Here's how the part is built. I have some questions about the finished solid (model axes, mm). Face numbers are marked on the shaded views. A direction names the side the tool comes from. Round coordinates to 2 decimals unless told otherwise and drop trailing zeros. Write each loop counter-clockwise with the first axis right and the second up, starting at its lowest first coordinate (ties: lowest second). Pieces come first, ordered by that corner, then holes. Notation, with made-up numbers: (82.25, 30) -> (126.25, 30) arc R9 ccw to (126.25, 39) -> close; hole circle Ø1 at (36, 64). An arc over 180 degrees is marked (long way). Put each result on its own line as item: value. Start each with the question number.
1. Suppose I cut it at D-D (z = 27). Count the separate pieces of the cut face and the enclosed holes in it, then the cut area to 3 significant figures.
2. Which directions (+Z, -Z, +X, -X, +Y, -Y) give clear straight access to the entire face, cutting with the end or side of a thin tool? Please do the marked faces 1 and 2.
3. Suppose I cut it at C-C (z = 7). Please give me the cut outline in (x, y), then the cut area to 3 significant figures.
4. Suppose I cut it at A-A (y = 0). Please give me the cut outline in (x, z), then the cut area to 3 significant figures.
5. For pin 1 (1.4 mm diameter, centred on x = -42, z = 27, fed in from +Y); pin 2 (1.6 mm diameter, centred on y = 12.5, z = 1, fed in from +X); pin 3 (1.6 mm diameter, centred on x = 54.5, z = 13, fed in from -Y), each with a flat end and sliding along its axis, tell me the tip position at first contact or that it passes through.
6. We'd pull the mould along X, two halves only. Please class the marked faces 3, 4 and 5: +X half, -X half, draft (parallel to the pull), parting line (faces both ways), or undercut.
7. Suppose I cut it at B-B (x = 0). Please give me the cut outline in (y, z).
8. I need wall thicknesses on probe 1 along Z at (x, y) = (34, 21); probe 2 along Z at (x, y) = (13, 24.5); probe 3 along Y at (x, z) = (-26, 12). Which ranges of each line are inside material? Lowest first, please. Write a range as from..to.
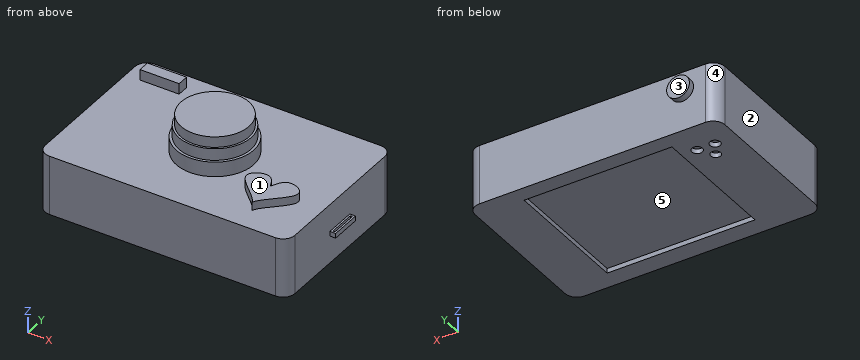
```python
from build123d import *

# Parameters (mm, degrees)
F0_W      = 106.945887208
F0_H      = 70.1787695289
F1_DEPTH  = 25.4
F2_R      = 16.5647442007
F3_DEPTH  = 6.35
F4_R      = 15.4514430259
F4_R_2    = 14.5768166451
F5_DEPTH  = 5.08
F6_W      = 16.7820453644
F6_H      = 4.9917921424
F7_DEPTH  = 4.572
F9_DEPTH  = 3.556
F10_R     = 4.8749560022
F11_DEPTH = 2.794
F12_R     = 5.08
F15_W     = 2.4653045057
F15_H     = 13.2586471736
F15_W_2   = 0.8905041559
F15_H_2   = 11.6838468239
F16_DEPTH = 1.016
F17_W     = 63.2937094197
F17_H     = 55.5002773181
F17_R     = 2.1212827151
F17_R_2   = 2.2190878442
F17_R_3   = 2.2757544949
F18_DEPTH = 2
F19_DEPTH = 9.652


with BuildPart() as f1:
    # F0 (on Top) → F1 (new body)
    with BuildSketch(Plane.XY):
        Rectangle(F0_W, F0_H)
    extrude(amount=F1_DEPTH)

    # F2 (on face) → F3 (join)
    with BuildSketch(Plane.XY.offset(25.4)):
        Circle(F2_R)
    extrude(amount=F3_DEPTH)

    # F4 (on face) → F5 (join)
    with BuildSketch(Plane.XY.offset(31.75)):
        Circle(F4_R)
        Circle(F4_R_2, mode=Mode.SUBTRACT)
    extrude(amount=F5_DEPTH)

    # F6 (on face) → F7 (join)
    with BuildSketch(Plane.XY.offset(25.4)):
        with Locations((-38.8989336789, 26.1253975332)):
            Rectangle(F6_W, F6_H)
    extrude(amount=F7_DEPTH)

    # F8 (on face) → F9 (join)
    with BuildSketch(Plane.XY.offset(25.4)):
        with BuildLine():
            add(Edge.make_bspline(
                [(31.8442881107, -12.6362098381), (32.9562300538, -10.0665577137), (35.221941382, -4.8305919654), (48.841003928, -11.6298962751), (33.3513436417, -20.9799528384), (31.8442881107, -24.8728917222)],
                knots=[0, 0, 0, 0, 0.1573778113, 0.3206756361, 0.533694036, 0.533694036, 0.533694036, 0.533694036], degree=3))
            add(Edge.make_bspline(
                [(31.8442881107, -12.6362098381), (30.7323461677, -10.0665577137), (28.4666348395, -4.8305919654), (14.8475722934, -11.6298962751), (30.3372325798, -20.9799528384), (31.8442881107, -24.8728917222)],
                knots=[0, 0, 0, 0, 0.1573778113, 0.3206756361, 0.533694036, 0.533694036, 0.533694036, 0.533694036], degree=3))
        make_face()
    extrude(amount=F9_DEPTH)

    # F10 (on face) → F11 (join)
    with BuildSketch(Plane(origin=(0, 35.0893847644, 0), x_dir=(-1, 0, 0), z_dir=(0, 1, 0))):
        with Locations((38.4255424142, 17.5938177854)):
            Circle(F10_R)
    extrude(amount=F11_DEPTH)

    # F12
    f12_edges = [f1.edges().sort_by_distance(p)[0] for p in [
        (53.472944, 35.089385, 12.7),
        (53.472944, -35.089385, 12.7),
        (-53.472944, 35.089385, 12.7),
        (-53.472944, -35.089385, 12.7),
    ]]
    fillet(f12_edges, radius=F12_R)

    # F15 (on plane+point) → F16 (join, symmetric)
    with BuildSketch(Plane.XY.offset(12.7)):
        with Locations((54.7055958568, 0)):
            Rectangle(F15_W, F15_H)
        with Locations((54.7055958568, 0)):
            Rectangle(F15_W_2, F15_H_2, mode=Mode.SUBTRACT)
    extrude(amount=F16_DEPTH, both=True)

    # F17 (on Top) → F18 (cut)
    with BuildSketch(Plane.XY):
        with Locations((1.9618016668, 0.582842622)):
            Rectangle(F17_W, F17_H)
        with Locations((-40.4380485415, 15.8517025411)):
            Circle(F17_R)
        with Locations((-43.9564026892, 21.7156279832)):
            Circle(F17_R_2)
        with Locations((-36.268144846, 21.7156279832)):
            Circle(F17_R_3)
    extrude(amount=F18_DEPTH, mode=Mode.SUBTRACT)

    # F19 (add): a face of the model
    f19_faces = [f1.faces().sort_by_distance(p)[0] for p in [
        (0, 0, 31.75),
    ]]
    extrude(f19_faces, amount=F19_DEPTH)


solid = f1.part
```
Verdict:
1. separate pieces: 3
1. enclosed holes: 0
1. area: 1,170 mm^2
2. face 1: +Z, +X, +Y, -Y
2. face 2: +Z, -Z, -X, +Y, -Y
3. outline: (-53.47, -30.01) arc R5.08 ccw to (-48.39, -35.09) -> (48.39, -35.09) arc R5.08 ccw to (53.47, -30.01) -> (53.47, 30.01) arc R5.08 ccw to (48.39, 35.09) -> (-48.39, 35.09) arc R5.08 ccw to (-53.47, 30.01) -> close
3. area: 7,480 mm^2
4. outline: (-53.47, 0) -> (-29.69, 0) -> (-29.69, 2) -> (33.61, 2) -> (33.61, 0) -> (53.47, 0) -> (53.47, 11.68) -> (54.26, 11.68) -> (54.26, 13.72) -> (53.47, 13.72) -> (53.47, 25.4) -> (16.56, 25.4) -> (16.56, 31.75) -> (15.45, 31.75) -> (15.45, 36.83) -> (14.58, 36.83) -> (14.58, 41.4) -> (-14.58, 41.4) -> (-14.58, 36.83) -> (-15.45, 36.83) -> (-15.45, 31.75) -> (-16.56, 31.75) -> (-16.56, 25.4) -> (-53.47, 25.4) -> close; (55.15, 11.68) -> (55.94, 11.68) -> (55.94, 13.72) -> (55.15, 13.72) -> close
4. area: 3,090 mm^2
5. pin 1: stops at y = 28.62
5. pin 2: stops at x = 53.47
5. pin 3: stops at y = -6.63
6. face 3: draft
6. face 4: -X half
6. face 5: undercut
7. outline: (-35.09, 0) -> (-27.17, 0) -> (-27.17, 2) -> (28.33, 2) -> (28.33, 0) -> (35.09, 0) -> (35.09, 25.4) -> (16.56, 25.4) -> (16.56, 31.75) -> (15.45, 31.75) -> (15.45, 36.83) -> (14.58, 36.83) -> (14.58, 41.4) -> (-14.58, 41.4) -> (-14.58, 36.83) -> (-15.45, 36.83) -> (-15.45, 31.75) -> (-16.56, 31.75) -> (-16.56, 25.4) -> (-35.09, 25.4) -> close
8. probe 1: z = 0..25.4
8. probe 2: z = 2..25.4
8. probe 3: y = -35.09..35.09
